The listing builds one solid part. Answer for the finished solid, in the listing's coordinates (mm). A direction names the side the tool comes from. Give positions to 0.01 mm unless a question says otherwise; leave off trailing zeros. One line per question, with ' | ' between items. Start each with the question number.
1. Find the intervals of material crossed by L1, parallel to Z at x = 38, y = -1; L2, parallel to Z at x = 4, y = -0.25; L3, parallel to X at y = -2.25, z = 10, in increasing order. Write a range as from..to.
2. Given P1, Ø6, axis at x = 54, z = 1.5, coming from the +Y side; P2, Ø2, axis at y = -1.5, z = 7, coming from the +X side; P3, Ø3, axis at y = -1, z = 15.5, coming from the +X side; P4, Ø1.8, axis at x = 54.67, z = 14.2, coming from the -Y side, each flat-ended and moving along its own axis, determine where each tip first touches the part or whether it passes through.
3. A cutting plane is placed at A-A (y = 0.75). State how many separate pieces and enclosed holes the cut face has, then the cut area to 3 significant figures.
4. For faces 1 (the face through (55, -2.25, 2)), 2 (the face through (55, 2.25, 2)), 3 (the face through (52.965, -0.031, 3.154)), determine the directions among +Z, -Z, +X, -X, +Y, -Y from which every point of the face is accessible in a straight line to the end or side of a thin tool.
5. The mould has two halves that part along X. Classify faces 4 (the face through (35.23, -0.05, -29.61)), 5 (the face through (57.28, -0.03, 0.98)), 6 (the face through (41.4, -3.5, 12)): +X half, -X half, draft (parallel to the pull), parting line (faces both ways), or undercut.
```python
from build123d import *

# Parameters (mm, degrees)
F0_R     = 1
F1_DEPTH = 3.5
F2_DEPTH = 2.25


# Not quite as in the source:
# - a feature names something its author has since deleted; it is built from what else it names


with BuildPart() as f1:
    # F0 (on Front) → F1 (new body, symmetric)
    with BuildSketch(Plane.XZ):
        with BuildLine():
            Line((62.29, 21.44), (0, 21.44))
            Line((0, 21.44), (0, 3.7288318854))
            Line((0, 3.7288318854), (6.67, 3.7288318854))
            Line((6.67, 3.7288318854), (6.67, 12.7888318854))
            add(Edge.make_bspline(
                [(6.67, 12.7888318854), (20.3660801053, 23.045424372), (38.400747317, 13.8677307047), (52.300490874, 6.170732399)],
                knots=[0, 0, 0, 0, 46.1079270648, 46.1079270648, 46.1079270648, 46.1079270648], degree=3))
            Line((52.300490874, 6.170732399), (53.4860821652, 5.5017437759))
            Line((53.4860821652, 5.5017437759), (57.9021407774, 2.7602773683))
            Line((57.9021407774, 2.7602773683), (58.3288028571, 2.49540775))
            add(Edge.make_bspline(
                [(34.304166128, -27.3203667793), (39.4049563141, -26.0173317216), (55.1670315062, -16.4703750294), (59.0722335282, -0.2752133185), (58.3288028571, 2.49540775)],
                knots=[0, 0, 0, 0, 0.5353864124, 1, 1, 1, 1], degree=3))
            Line((34.304166128, -27.3203667793), (36.1752310606, -31.9570807038))
            ThreePointArc((36.1752310606, -31.9570807038), (59.6028549739, -10.3302859108), (62.29, 21.44))
        make_face()
        with Locations((37.5891347185, -28.6906498222)):
            Circle(F0_R, mode=Mode.SUBTRACT)
        with Locations((3.4974589944, 6.6614318639)):
            Circle(F0_R, mode=Mode.SUBTRACT)
        with Locations((3.4974589944, 17.5246726722)):
            Circle(F0_R, mode=Mode.SUBTRACT)
        with Locations((54.66741696, 14.1964312643)):
            Circle(F0_R, mode=Mode.SUBTRACT)
    extrude(amount=F1_DEPTH, both=True)

    # F0 (on Front) → F2 (join, symmetric)
    with BuildSketch(Plane.XZ):
        Polygon((56.6776084413, -0.7441981102), (57.9021407774, 2.7602773683), (53.4860821652, 5.5017437759), (52.4294775853, 0.7401819728), align=None)
    extrude(amount=F2_DEPTH, both=True)


solid = f1.part
```
Determined:
1) L1: -31.19..-29.6, -27.78..-25.97, 13.31..21.44 | L2: 3.73..5.8, 7.53..16.66, 18.39..21.44 | L3: 0..6.67, 45.14..64.07
2) P1: y = 2.25 | P2: x = 64.07 | P3: x = 63.8 | P4: through
3) separate pieces: 1 | enclosed holes: 4 | area: 856 mm2
4) face 1: -Y | face 2: +Y | face 3: +Y, -Y
5) face 4: -X half | face 5: undercut | face 6: draft
